Study the drawing (mm; zero at the part's minimum x, y, z) and answer. A direction names the side the tool comes from. Coordinates: 2 decimals unless noted, no trailing zeros. Write each loop counter-clockwise with the first axis right and the second up, starting at its lowest first coordinate (ties: lowest second). Pieces come first, ordered by that corner, then holes. Notation, with made-up numbers: (16, 72) -> (54, 72) arc R18 cw to (54, 86) -> close; hole circle Ø7 at (-39, -4.75). An arc over 180 degrees is marked (long way). Answer in a Markdown table with one row per item. Add a question column.
Item 1: Section A-A on z = 5 is taken. Write down the section's boundary in (x, y).
Item 2: Section C-C on y = 30 is taken. Write down the section's boundary in (x, z).
Item 3: Given pin 1 Ø23 at (x, y) = (70, 44) entering from +Z; pin 2 Ø20.5 at (y, z) = (17.5, 11.5) entering from +X; pin 3 Ø7.5 at (x, z) = (43.5, 20.5) entering from +Y, each flat-ended and moving along its own axis, determine where each tip first touches the part or whether it passes through.
Item 4: Which of the six approach directions +Z, -Z, +X, -X, +Y, -Y give full straight-line access (tool end or side, diameter ignored) to the marked faces 1, 2 and 3?
Item 5: Section B-B on x = 120.5 is taken. Write down the section's boundary in (y, z), then the cut area to 3 significant figures.
Item 6: Straight lines are drawn through the part: line 1 (Y direction, x = 55, z = 26); line 2 (X direction, y = 9, z = 26). For each, find the intervals that lie inside material, in ascending order. Write a range as from..to.
Item 7: Section D-D on x = 68 is taken. Write down the section's boundary in (y, z), then the cut area to 3 significant figures.
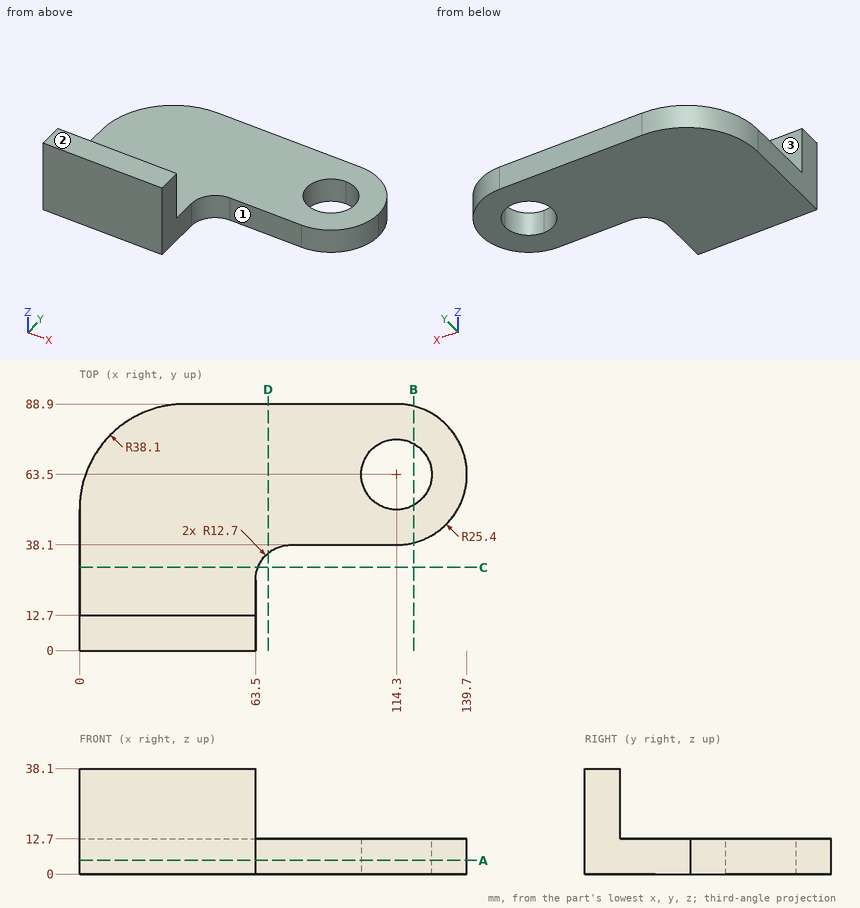
Results below:
| question | item | result |
|---|---|---|
| 1 | outline | (0, 0) -> (63.5, 0) -> (63.5, 25.4) arc R12.7 cw to (76.2, 38.1) -> (114.3, 38.1) arc R25.4 ccw to (114.3, 88.9) -> (38.1, 88.9) arc R38.1 ccw to (0, 50.8) -> close; hole circle Ø25.4 at (114.3, 63.5) |
| 2 | outline | (0, 0) -> (64.36, 0) -> (64.36, 12.7) -> (0, 12.7) -> close |
| 3 | pin 1 | stops at z = 12.7 |
| 3 | pin 2 | stops at x = 63.72 |
| 3 | pin 3 | stops at y = 12.7 |
| 4 | face 1 | +Z, -Z, +X, -Y |
| 4 | face 2 | +Z, +X, -X, +Y, -Y |
| 4 | face 3 | +Z, +X, -X, +Y |
| 5 | outline | (38.87, 0) -> (52.42, 0) -> (52.42, 12.7) -> (38.87, 12.7) -> close; (74.58, 0) -> (88.13, 0) -> (88.13, 12.7) -> (74.58, 12.7) -> close |
| 5 | area | 344 mm2 |
| 6 | line 1 | y = 0..12.7 |
| 6 | line 2 | x = 0..63.5 |
| 7 | outline | (35.1, 0) -> (88.9, 0) -> (88.9, 12.7) -> (35.1, 12.7) -> close |
| 7 | area | 683 mm2 |
